Verification items for this drawing (mm, ordinates from the low corner). Coordinates: 2 decimals unless noted, no trailing zeros. Write each loop counter-clockwise with the first axis right and the second up, starting at its lowest first coordinate (ties: lowest second). Pieces come first, ordered by that corner, then holes. Notation, with made-up numbers: (45, 28) -> (101, 28) arc R17 ccw to (101, 34) -> close; hole circle Ø7 at (-24.75, 48.5). An arc over 180 degrees is marked (long way). One line per question, with ' | ' between items.
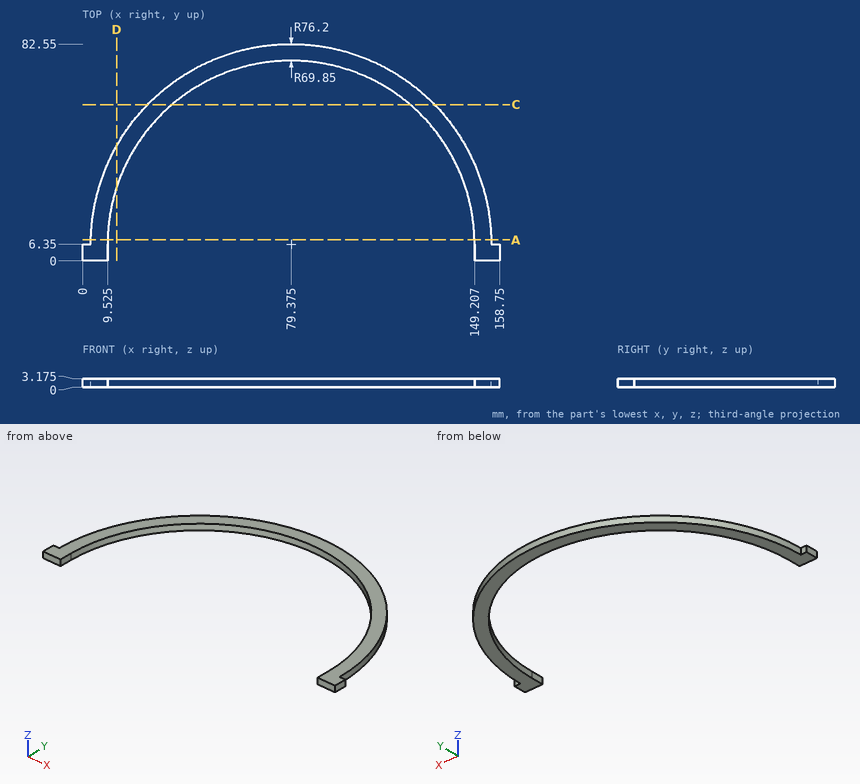
(1) Cross-section at D-D (x = 13). Record the cut outline in (y, z) (1 decimal).
Answers below:
outline: (28.1, 0) -> (43.8, 0) -> (43.8, 3.2) -> (28.1, 3.2) -> close
(2) Cross-section at C-C (y = 59.5). Record the cut outline in (x, z) (1 decimal).
Answers below:
outline: (24.8, 0) -> (34.1, 0) -> (34.1, 3.2) -> (24.8, 3.2) -> close; (124.7, 0) -> (134, 0) -> (134, 3.2) -> (124.7, 3.2) -> close
(3) Material ranges on line 1 (Y direction, x = 79, z = 2.5); line 2 (X direction, y = 63, z = 0.45) (1 decimal); line 3 (X direction, y = 37.5, z = 1.6) (1 decimal), recorded low to high.
Answers below:
line 1: y = 76.2 to 82.55 | line 2: x = 28.4 to 38.5, 120.2 to 130.3 | line 3: x = 9.8 to 16.9, 141.9 to 148.9
(4) Cross-section at A-A (y = 8). Record the cut outline in (x, z) (1 decimal).
Answers below:
outline: (3.2, 0) -> (9.5, 0) -> (9.5, 3.2) -> (3.2, 3.2) -> close; (149.2, 0) -> (155.6, 0) -> (155.6, 3.2) -> (149.2, 3.2) -> close
(5) Depth check by flat-ended pin: P1, Ø1.5, axis at x = 81, z = 2, coming from the -Y side; P2, Ø1, axis at x = 2, z = 2.5, coming from the +Y side; P3, Ø1, axis at x = 28.5, z = 2.5, coming from the -Y side (1 decimal). Enter the tip coordinate at first touch or a pass-through.
Answers below:
P1: stops at y = 76.16 | P2: stops at y = 6.35 | P3: stops at y = 53.7
